Print and shaded views of the part. All mm, measured from the part's lowest x, y and z. A direction names the side the tool comes from. Round coordinates to 2 decimals unless told otherwise and drop trailing zeros. Order: outer loops, then holes, each group sorted by start corner. A loop starts at its lowest first (then second) coordinate and runs counter-clockwise, first axis right, second up. Notation, with made-up numbers: (-32, -14.75) - (-27, -14.75) arc R6 cw to (-27, -5.75) - close; hole circle Ø6 at (-19.75, 51). An arc over 180 degrees is marked (long way). Return JSON: item names as keys, results as strings. Group by question number.
Item 1: Saw through at A-A on z = 8. List the corners of the cut face in (x, y), and give its area (3 significant figures).
Item 2: Tool access for the marked faces 1 and 2: list every direction of +Z, -Z, +X, -X, +Y, -Y with a clear straight run to the whole face (end or side of a thin tool).
Item 3: Saw through at C-C on z = 20. List the corners of the cut face in (x, y).
Item 4: Saw through at B-B on x = 20. List the corners of the cut face in (y, z), and give its area (3 significant figures).
Item 5: Saw through at D-D on y = 46. List the corners of the cut face in (x, z).
Item 6: Probe probe 1 along Y at (x, z) = (26, 32.5); probe 2 along Y at (x, z) = (25.5, 5); probe 3 along Z at (x, y) = (36, 67.5). List the from-to ranges inside material, lowest first.
Item 7: Drop flat-ended pins along their axis: pin 1 (8 mm diameter, centred on y = 63.5, z = 4.5, fed in from +X); pin 2 (10 mm diameter, centred on x = 4.5, y = 64, fed in from +Z); pin 3 (1.5 mm diameter, centred on y = 9.5, z = 16.5, fed in from +X); pin 4 (9 mm diameter, centred on x = 27, z = 27, fed in from -Y). Give the stop position or say it passes through.
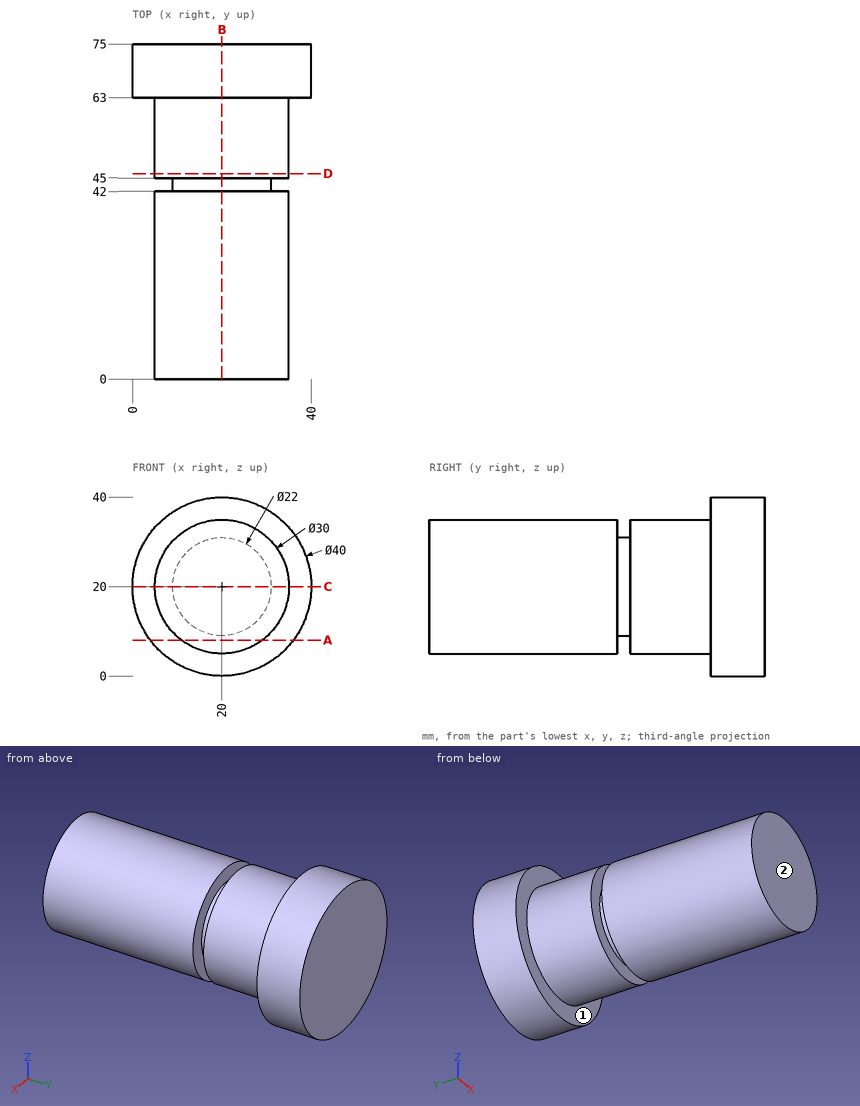
Filled in:
{
 "1": {"outline": "(4, 63) - (11, 63) - (11, 45) - (29, 45) - (29, 63) - (36, 63) - (36, 75) - (4, 75) - close; (11, 0) - (29, 0) - (29, 42) - (11, 42) - close", "area": "1,460 mm^2"},
 "2": {"face 1": "-Y", "face 2": "+Z, -Z, +X, -X, -Y"},
 "3": {"outline": "(0, 63) - (5, 63) - (5, 45) - (9, 45) - (9, 42) - (5, 42) - (5, 0) - (35, 0) - (35, 42) - (31, 42) - (31, 45) - (35, 45) - (35, 63) - (40, 63) - (40, 75) - (0, 75) - close"},
 "4": {"outline": "(0, 5) - (42, 5) - (42, 9) - (45, 9) - (45, 5) - (63, 5) - (63, 0) - (75, 0) - (75, 40) - (63, 40) - (63, 35) - (45, 35) - (45, 31) - (42, 31) - (42, 35) - (0, 35) - close", "area": "2,350 mm^2"},
 "5": {"outline": "circle Ø30 at (20, 20)"},
 "6": {"probe 1": "y = 0 to 42, 45 to 75", "probe 2": "y = 63 to 75", "probe 3": "z = 8 to 32"},
 "7": {"pin 1": "stops at x = 36.36", "pin 2": "stops at z = 37.02", "pin 3": "stops at x = 34.75", "pin 4": "stops at y = 0"}
}
